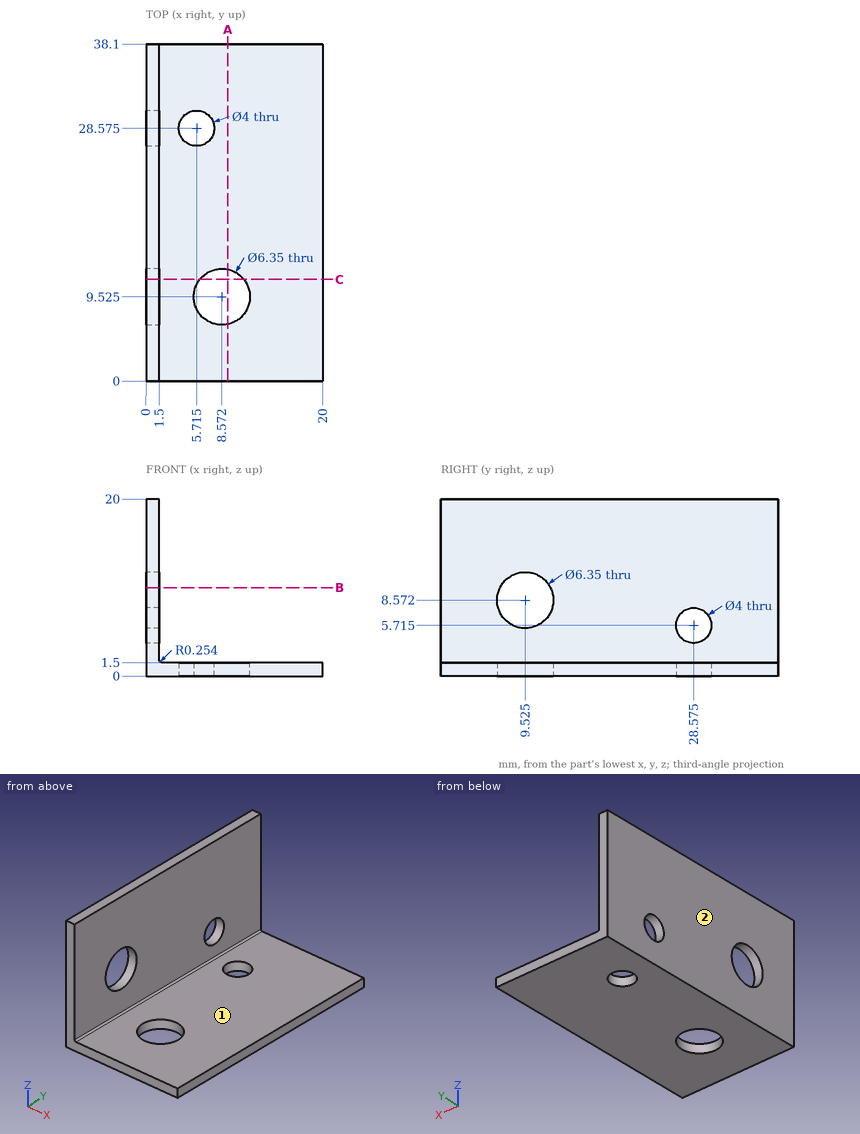
Answer from the drawing. Dimensions are ordinates in mm from the lowest x, y and z of the part. A direction names the side the tool comes from. Coordinates: 2 decimals unless noted, no trailing zeros. Write each loop counter-clockwise with the first axis right and the second up, starting at its lowest first coordinate (ties: lowest second). Pieces come first, ordered by that corner, then holes. Notation, with made-up numbers: (1, 43.25) - (12, 43.25) arc R20 ccw to (12, 79.25) - close; hole circle Ø9 at (-17, 25.5). An arc over 180 degrees is marked (long way). One line per question, with ' | ' between items.
Q1. Find section A-A, the plane x = 9.25. Write down the section's boundary in (y, z).
Result set:
outline: (0, 0) - (6.42, 0) - (6.42, 1.5) - (0, 1.5) - close; (12.63, 0) - (38.1, 0) - (38.1, 1.5) - (12.63, 1.5) - close
Q2. Find section B-B, the plane z = 10. Write down the section's boundary in (x, y).
Result set:
outline: (0, 0) - (1.5, 0) - (1.5, 6.69) - (0, 6.69) - close; (0, 12.36) - (1.5, 12.36) - (1.5, 38.1) - (0, 38.1) - close
Q3. For the marked faces 1 and 2, determine the directions among +Z, -Z, +X, -X, +Y, -Y from which every point of the face is accessible in a straight line to the end or side of a thin tool.
Result set:
face 1: +Z, +X, +Y, -Y | face 2: +Z, -Z, -X, +Y, -Y
Q4. Find section C-C, the plane y = 11.5. State how many separate pieces and enclosed holes the cut face has.
Result set:
separate pieces: 3 | enclosed holes: 0
Q5. Consider L1, parallel to Z at x = 12.5, y = 32. Determine where the line is inside the solid, lowest interval first. Write a range as [from, to].
Result set:
L1: [0, 1.5]
Q6. Each of these flat-tipped pins is pushed along its axis until it touches: P1, Ø7.5, axis at x = 8.57, y = 9.52, coming from the -Z side; P2, Ø6, axis at y = 27, z = 12.5, coming from the +X side; P3, Ø9, axis at x = 7.5, y = 28.5, coming from the +Z side. Where does it stop, or does it pass through?
Result set:
P1: z = 0 | P2: x = 1.5 | P3: z = 1.5
